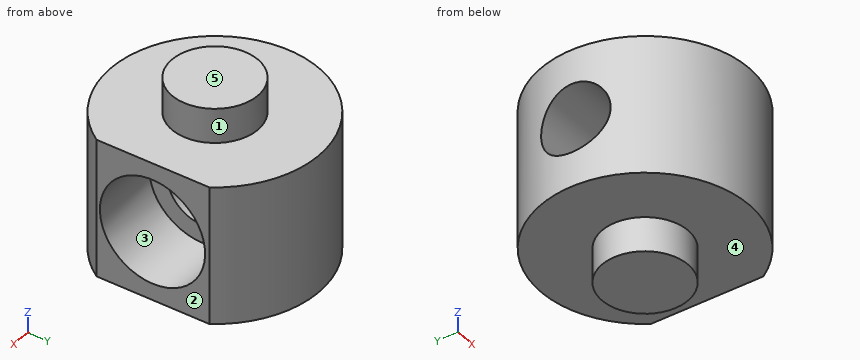
```python
from build123d import *

# Parameters (mm, degrees)
CUT_EXTRUDE1_DEPTH = 12.7
SKETCH3_R          = 3.175
CUT_EXTRUDE2_DEPTH = 28.582400204
SKETCH3_3_R        = 4.826
SKETCH3_3_R_2      = 3.175
CUT_EXTRUDE3_DEPTH = 6.35


with BuildPart() as part:
    # Sketch1 → Revolve1 (revolve)
    with BuildSketch(Plane(origin=(0, 0, 0), x_dir=(1, 0, 0), z_dir=(0, 1, 0))):
        Polygon((0, 0), (3.937, 0), (3.937, -3.175), (9.525, -3.175), (9.525, -15.875), (3.937, -15.875), (3.937, -19.05), (0, -19.05), align=None)
    revolve(axis=Axis((0, 0, 19.05), (0, 0, -1)))

    # Sketch2 → Cut-Extrude1 (cut)
    with BuildSketch(Plane.XY.offset(15.875)):
        Polygon((8.001, 60.908660379), (8.001, 5.168135447), (8.001, 0), (8.001, -5.168135447), (8.001, -60.908660379), (119.482049864, -60.908660379), (119.482049864, 60.908660379), align=None)
    extrude(amount=-CUT_EXTRUDE1_DEPTH, mode=Mode.SUBTRACT)

    # Sketch3 → Cut-Extrude2 (cut, through all)
    with BuildSketch(Plane(origin=(8.001, 0, 0), x_dir=(0, 0, -1), z_dir=(1, 0, 0))):
        with Locations((-9.525, -0.038864553)):
            Circle(SKETCH3_R)
    extrude(amount=-CUT_EXTRUDE2_DEPTH, mode=Mode.SUBTRACT)

    # Sketch3<3> → Cut-Extrude3 (cut)
    with BuildSketch(Plane(origin=(8.001, 0, 0), x_dir=(0, 0, -1), z_dir=(1, 0, 0))):
        with Locations((-9.525, -0.038864553)):
            Circle(SKETCH3_3_R)
        with Locations((-9.525, -0.038864553)):
            Circle(SKETCH3_3_R_2, mode=Mode.SUBTRACT)
    extrude(amount=-CUT_EXTRUDE3_DEPTH, mode=Mode.SUBTRACT)


solid = part.part
```
Design review of the part built by this model. Coordinates are the model's own, in mm. Face numbers are marked on the shaded views. A direction names the side the tool comes from. Round coordinates to 2 decimals unless told otherwise and drop trailing zeros. Write each loop counter-clockwise with the first axis right and the second up, starting at its lowest first coordinate (ties: lowest second). Pieces come first, ordered by that corner, then holes.
Item 1: Clearance check with flat-ended pins moving along their axes: pin 1 Ø1.5 at (x, y) = (1, -6.5) entering from -Z (3 decimals); pin 2 Ø4 at (y, z) = (3, 13) entering from -X; pin 3 Ø2 at (x, y) = (-6.5, 5) entering from +Z (3 decimals). State where each tip first meets the part, or that it passes through.
Item 2: We need section D-D on z = 8. Write out the cut boundary in (x, y) (3 decimals), and give its area (3 significant figures).
Item 3: We need section B-B on z = 12.25. Write out the cut boundary in (x, y) (3 decimals), and give its area (3 significant figures).
Item 4: We need section A-A on y = 1.75. Write out the cut boundary in (x, z) (3 decimals), and give its area (3 significant figures).
Item 5: For probe 1 along Y at (x, z) = (-8, 3.25); probe 2 along Z at (x, y) = (-4.25, 7) (3 decimals); probe 3 along Z at (x, y) = (-7.25, 0.75) (3 decimals), list the stretches that pass through material, from the lowest coordinate up.
Item 6: The part is to be moulded in two halves that separate along Y. For the marked faces 1, 2 and 3, say which applies: +Y half, -Y half, draft (parallel to the pull), parting line (faces both ways), or undercut.
Item 7: For the marked faces 4 and 5, list the 3-axis set-ups (+Z, -Z, +X, -X, +Y, -Y) from which the entire face can be reached by the end or side of a thin tool; tool diameter is ignored.
Item 8: We need section C-C on x = 0. Write out the cut boundary in (y, z) (3 decimals).
Returned:
1. pin 1: stops at z = 3.175
1. pin 2: stops at x = -9.47
1. pin 3: stops at z = 15.875
2. outline: (-9.121, 2.746) - (1.651, 2.746) - (1.651, 4.54) - (8.001, 4.54) - (8.001, 5.168) arc R9.525 ccw to start; (-9.097, -2.824) arc R9.525 ccw to (8.001, -5.168) - (8.001, -4.618) - (1.651, -4.618) - (1.651, -2.824) - close
2. area: 155 mm2
3. outline: (-9.391, 1.591) - (1.651, 1.591) - (1.651, 3.944) - (8.001, 3.944) - (8.001, 5.168) arc R9.525 ccw to start; (-9.378, -1.668) arc R9.525 ccw to (8.001, -5.168) - (8.001, -4.022) - (1.651, -4.022) - (1.651, -1.668) - close
3. area: 187 mm2
4. outline: (-9.363, 3.175) - (-3.527, 3.175) - (-3.527, 0) - (3.527, 0) - (3.527, 3.175) - (8.001, 3.175) - (8.001, 5.043) - (1.651, 5.043) - (1.651, 6.902) - (-9.363, 6.902) - close; (-9.363, 12.148) - (1.651, 12.148) - (1.651, 14.007) - (8.001, 14.007) - (8.001, 15.875) - (3.527, 15.875) - (3.527, 19.05) - (-3.527, 19.05) - (-3.527, 15.875) - (-9.363, 15.875) - close
4. area: 151 mm2
5. probe 1: y = -5.17 to 5.17
5. probe 2: z = 3.175 to 15.875
5. probe 3: z = 3.175 to 6.45, 12.6 to 15.875
6. face 1: parting line
6. face 2: draft
6. face 3: undercut
7. face 4: -Z
7. face 5: +Z, +X, -X, +Y, -Y
8. outline: (-9.525, 3.175) - (-3.937, 3.175) - (-3.937, 0) - (3.937, 0) - (3.937, 3.175) - (9.525, 3.175) - (9.525, 15.875) - (3.937, 15.875) - (3.937, 19.05) - (-3.937, 19.05) - (-3.937, 15.875) - (-9.525, 15.875) - close; hole circle Ø6.35 at (-0.039, 9.525)
